Read the model definition and answer for the solid it produces. Units are mm, in the model's axes. Face numbers are marked on the shaded views. A direction names the side the tool comes from. Round coordinates to 2 decimals unless told otherwise and drop trailing zeros. Loops run counter-clockwise (first coordinate to the right, second up) from the corner with the lowest first, then second, coordinate; pieces in that order, holes last. Notation, with made-up numbers: (22, 35) - (72, 35) arc R26 cw to (72, 71) - close; hole circle Ø4 at (51.5, 25). An arc over 180 degrees is marked (long way). Use CSV: the item, a comma, the result in double quotes. Start each with the question number.
1. A tool of negligible diameter and unlimited length cuts with its end or side. For the marked faces 1 and 2, from which of +Z, -Z, +X, -X, +Y, -Y can it reach the whole face along a straight path? Write none if from no direction.
2. Find section B-B (x = 23). Give the vertices of the cut face in (y, z) (3 decimals), and give its area (3 significant figures).
3. Find section D-D (z = -16). Give the vertices of the cut face in (x, y) (3 decimals), and give its area (3 significant figures).
4. Given pin 1 Ø1.5 at (y, z) = (-5.5, -28) entering from +X (3 decimals); pin 2 Ø8 at (x, y) = (7.5, 0.5) entering from +Z; pin 3 Ø2 at (y, z) = (-8, -31) entering from -X; pin 4 Ø1.6 at (y, z) = (-1, -45) entering from -X, each flat-ended and moving along its own axis, determine where each tip first touches the part or whether it passes through.
5. Find section C-C (z = -1.5). Give the vertices of the cut face in (x, y) (3 decimals).
6. Consider line 1 along X through (y, z) = (-0.25, -40) (3 decimals); line 2 along Z through (x, y) = (40, -1) (3 decimals); line 3 along Y through (x, z) = (1, -6) (3 decimals). Determine where each line is inside the solid, lowest interval first.
7. Find section A-A (y = 4.25). Give the vertices of the cut face in (x, z) (3 decimals), and give its area (3 significant figures).
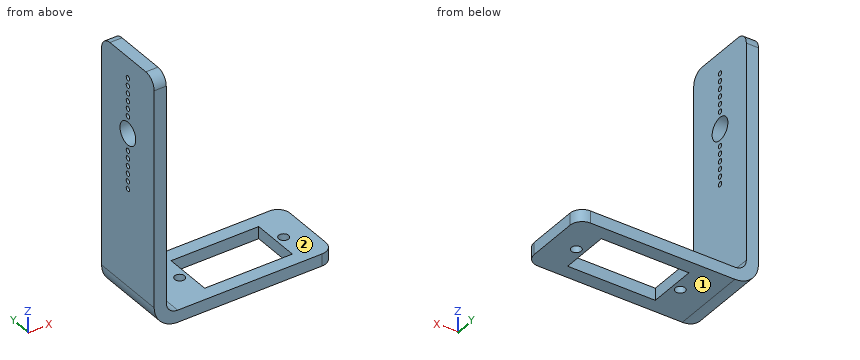
Autodesk Inventor part; units mm, degrees
ref_plane "YZ Plane" through (0, 0, 0) normal (1, 0, 0) x (0, 1, 0)
ref_plane "XZ Plane" through (0, 0, 0) normal (0, 1, 0) x (-1, 0, 0)
ref_plane "XY Plane" through (0, 0, 0) normal (0, 0, 1) x (1, 0, 0)
sketch "Sketch1" plane through (0, 0, 0) normal (1, 0, 0) x (0, 1, 0)
  circle A0 centre (0, 0) radius 2.5 construction
  circle A1 centre (0, 0) radius 3
  line L0 (0, 0) -> (0, -32.9) construction
  line L1 (-10, -85.8) -> (10, -85.8)
  line L2 (10, -85.8) -> (10, 20)
  line L3 (10, 20) -> (-10, 20)
  line L4 (-10, 20) -> (-10, -85.8)
  line L5 (-10, -85.8) -> (10, 20) construction
  line L6 (10, -85.8) -> (-10, 20) construction
  circle A2 centre (0, 0) radius 4.5 construction
  circle A3 centre (0, -4.5) radius 0.625
  circle A4 centre (0, -6.5) radius 0.625
  circle A5 centre (0, -8.5) radius 0.625
  circle A6 centre (0, -10.5) radius 0.625
  circle A7 centre (0, -12.5) radius 0.625
  circle A8 centre (0, -14.5) radius 0.625
  circle A9 centre (0, 14.5) radius 0.625
  circle A10 centre (0, 12.5) radius 0.625
  circle A11 centre (0, 10.5) radius 0.625
  circle A12 centre (0, 8.5) radius 0.625
  circle A13 centre (0, 6.5) radius 0.625
  circle A14 centre (0, 4.5) radius 0.625
  line L7 (-6.4, -54.3) -> (6.4, -54.3)
  line L8 (6.4, -54.3) -> (6.4, -77.3)
  line L9 (6.4, -77.3) -> (-6.4, -77.3)
  line L10 (-6.4, -77.3) -> (-6.4, -54.3)
  line L11 (-6.4, -54.3) -> (6.4, -77.3) construction
  line L12 (6.4, -54.3) -> (-6.4, -77.3) construction
  circle A15 centre (0, -65.8) radius 13.65 construction
  circle A16 centre (0, -79.45) radius 1.3
  circle A17 centre (0, -52.15) radius 1.3
  dimension "d5" = 9
  dimension "d19" = 27.3
  dimension "d0" = 5
  dimension "d1" = 6
  dimension "d2" = 20
  dimension "d3" = 105.8
  dimension "d4" = 20
  dimension "d6" = 1.25
  dimension "d9" = 2
  dimension "d16" = 360
  dimension "d18" = 23
  dimension "d20" = 2.6
  dimension "d21" = 12.8
  dimension "d24" = 360
  dimension "d26" = 20
extrude "Extrusion1" add sketch "Sketch1" along normal blind 3.175
fillet "Fillet1" radius 3.175 4 edges at (1.5875, 10, 20) (1.5875, -10, 20) (1.5875, 10, -85.8) (1.5875, -10, -85.8)
sketch "Sketch2" plane through (3.175, 0, 0) normal (1, 0, 0) x (0, 0, -1)
  line L0 (82.625, 10) -> (-16.825, 10)
  line L1 (40, 10) -> (40, -10)
  line L2 (-16.825, -10) -> (82.625, -10)
  line L3 (-20, 6.825) -> (-20, -6.825)
  point P0 (0, 0)
  dimension "d30" = 60
bend part "Bend Part1" radius 3 angle 90 line through (3.175, 10, -40) along (0, -1, 0) centre toward (1, 0, 0) moving side (0, 0, -1) both sides no
properties part number "Topplate"
Filled sheet:
1,face 1,"-Z, +X, -X, +Y, -Y"
1,face 2,"+Z, +X, +Y, -Y"
2,outline,"(-10, -46.175) - (-6.4, -46.175) - (-6.4, -43) - (-10, -43) - close; (6.4, -46.175) - (10, -46.175) - (10, -43) - (6.4, -43) - close"
2,area,"22.9 mm²"
3,outline,"(0, -10) - (3.175, -10) - (3.175, 10) - (0, 10) - close"
3,area,"63.5 mm²"
4,pin 1,"stops at x = 3.175"
4,pin 2,"stops at z = -41.36"
4,pin 3,"stops at x = 0"
4,pin 4,"stops at x = 1.65"
5,outline,"(0, -10) - (3.175, -10) - (3.175, -2.598) - (0, -2.598) - close; (0, 2.598) - (3.175, 2.598) - (3.175, 10) - (0, 10) - close"
6,line 1,"x = 0 to 3.175"
6,line 2,"z = -46.175 to -43"
6,line 3,"y = -10 to -0.375, 0.375 to 10"
7,outline,"(0, -40) arc R6.175 ccw to (6.175, -46.175) - (15.763, -46.175) - (15.763, -43) - (6.175, -43) arc R3 cw to (3.175, -40) - (3.175, 20) - (0, 20) - close; (38.763, -46.175) - (47.263, -46.175) - (47.263, -43) - (38.763, -43) - close"
7,area,"271 mm²"
